Can you work these out from the model? Positions are in its coordinate system, mm. A direction names the side the tool comes from. Round coordinates to 2 decimals unless told otherwise and drop trailing zeros. Loops run counter-clockwise (first coordinate to the right, second up) from the corner with the lowest first, then second, coordinate; pieces in that order, holes last. Notation, with made-up numbers: (-21, 84.5) -> (6, 84.5) arc R3 cw to (6, 88.5) -> close; hole circle Ø11 at (74, -27). An arc over 180 degrees is marked (long way). Write each question's results on one line, items separated by ' | '.
from build123d import *

# Parameters (mm, degrees)
SKETCH1_R           = 1
SKETCH1_W           = 3
SKETCH1_H           = 5
BOSS_EXTRUDE1_DEPTH = 3


with BuildPart() as part:
    # Sketch1 → Boss-Extrude1 (new body)
    with BuildSketch(Plane.XY):
        with BuildLine():
            ThreePointArc((20, 38.729833462), (19.160374698, 38.936968749), (18.316467633, 39.125904029))
            Line((18.316467633, 39.125904029), (17.276909179, 34.235166026))
            Line((17.276909179, 34.235166026), (14.342466376, 34.858901098))
            Line((14.342466376, 34.858901098), (15.35860178, 39.639442314))
            ThreePointArc((15.35860178, 39.639442314), (12.685359142, 39.909758785), (10, 40))
            Line((10, 40), (10, 35))
            Line((10, 35), (7, 35))
            Line((7, 35), (7, 39.88734135))
            ThreePointArc((7, 39.88734135), (3.47428501, 39.464098164), (0, 38.729833462))
            Line((0, 38.729833462), (0, 0))
            Line((0, 0), (20, 0))
            Line((20, 0), (20, 38.729833462))
        make_face()
        with Locations((2.5, 2.5)):
            Circle(SKETCH1_R, mode=Mode.SUBTRACT)
        with Locations((2.5, 5.5)):
            Circle(SKETCH1_R, mode=Mode.SUBTRACT)
        with Locations((2.5, 8.5)):
            Circle(SKETCH1_R, mode=Mode.SUBTRACT)
        with Locations((5.5, 2.5)):
            Circle(SKETCH1_R, mode=Mode.SUBTRACT)
        with Locations((8.5, 2.5)):
            Circle(SKETCH1_R, mode=Mode.SUBTRACT)
        with Locations((5.5, 5.5)):
            Circle(SKETCH1_R, mode=Mode.SUBTRACT)
        with Locations((5.5, 8.5)):
            Circle(SKETCH1_R, mode=Mode.SUBTRACT)
        with Locations((8.5, 5.5)):
            Circle(SKETCH1_R, mode=Mode.SUBTRACT)
        with Locations((8.5, 8.5)):
            Circle(SKETCH1_R, mode=Mode.SUBTRACT)
        with Locations((2.5, 11.5)):
            Circle(SKETCH1_R, mode=Mode.SUBTRACT)
        with Locations((2.5, 14.5)):
            Circle(SKETCH1_R, mode=Mode.SUBTRACT)
        with Locations((2.5, 17.5)):
            Circle(SKETCH1_R, mode=Mode.SUBTRACT)
        with Locations((5.5, 11.5)):
            Circle(SKETCH1_R, mode=Mode.SUBTRACT)
        with Locations((5.5, 14.5)):
            Circle(SKETCH1_R, mode=Mode.SUBTRACT)
        with Locations((8.5, 11.5)):
            Circle(SKETCH1_R, mode=Mode.SUBTRACT)
        with Locations((8.5, 14.5)):
            Circle(SKETCH1_R, mode=Mode.SUBTRACT)
        with Locations((5.5, 17.5)):
            Circle(SKETCH1_R, mode=Mode.SUBTRACT)
        with Locations((8.5, 17.5)):
            Circle(SKETCH1_R, mode=Mode.SUBTRACT)
        with Locations((11.5, 2.5)):
            Circle(SKETCH1_R, mode=Mode.SUBTRACT)
        with Locations((14.5, 2.5)):
            Circle(SKETCH1_R, mode=Mode.SUBTRACT)
        with Locations((11.5, 5.5)):
            Circle(SKETCH1_R, mode=Mode.SUBTRACT)
        with Locations((11.5, 8.5)):
            Circle(SKETCH1_R, mode=Mode.SUBTRACT)
        with Locations((14.5, 5.5)):
            Circle(SKETCH1_R, mode=Mode.SUBTRACT)
        with Locations((14.5, 8.5)):
            Circle(SKETCH1_R, mode=Mode.SUBTRACT)
        with Locations((17.5, 2.5)):
            Circle(SKETCH1_R, mode=Mode.SUBTRACT)
        with Locations((17.5, 5.5)):
            Circle(SKETCH1_R, mode=Mode.SUBTRACT)
        with Locations((17.5, 8.5)):
            Circle(SKETCH1_R, mode=Mode.SUBTRACT)
        with Locations((11.5, 11.5)):
            Circle(SKETCH1_R, mode=Mode.SUBTRACT)
        with Locations((11.5, 14.5)):
            Circle(SKETCH1_R, mode=Mode.SUBTRACT)
        with Locations((14.5, 11.5)):
            Circle(SKETCH1_R, mode=Mode.SUBTRACT)
        with Locations((14.5, 14.5)):
            Circle(SKETCH1_R, mode=Mode.SUBTRACT)
        with Locations((11.5, 17.5)):
            Circle(SKETCH1_R, mode=Mode.SUBTRACT)
        with Locations((14.5, 17.5)):
            Circle(SKETCH1_R, mode=Mode.SUBTRACT)
        with Locations((17.5, 11.5)):
            Circle(SKETCH1_R, mode=Mode.SUBTRACT)
        with Locations((17.5, 14.5)):
            Circle(SKETCH1_R, mode=Mode.SUBTRACT)
        with Locations((17.5, 17.5)):
            Circle(SKETCH1_R, mode=Mode.SUBTRACT)
        with Locations((8.5, 22.5)):
            Rectangle(SKETCH1_W, SKETCH1_H, mode=Mode.SUBTRACT)
        Polygon((15.19779227, 24.453690018), (14.158233816, 19.562952015), (11.223791014, 20.186687087), (12.263349468, 25.077425091), align=None, mode=Mode.SUBTRACT)
    extrude(amount=BOSS_EXTRUDE1_DEPTH)


solid = part.part
1. If we section it at A-A (x = 8.5): State how many separate pieces and enclosed holes the cut face has, then the cut area to 3 significant figures.
Final values:
separate pieces: 8 | enclosed holes: 0 | area: 54.0 mm2
2. On a 3-axis mill with a long thin cutter (end or side, diameter ignored), from which of +Z, -Z, +X, -X, +Y, -Y can I reach the whole of each face in a straight line? I mean faces 1 (the face through (17.8, 36.7, 1.5)), 2 (the face through (8, 20, 1)). Say none if no direction works.
Final values:
face 1: +Z, -Z, +Y | face 2: +Z, -Z
3. Will this pin go through, and if not, where does the flat tip stop? pin 1 (1.5 mm diameter, centred on x = 5, z = 2, fed in from +Y).
Final values:
pin 1: y = 39.77
4. If we section it at D-D (y = 22.5): List the corners of the cut face in (x, z) for me.
Final values:
outline: (0, 0) -> (7, 0) -> (7, 3) -> (0, 3) -> close; (10, 0) -> (11.72, 0) -> (11.72, 3) -> (10, 3) -> close; (14.78, 0) -> (20, 0) -> (20, 3) -> (14.78, 3) -> close
5. If we section it at B-B (y = 5.5): List the corners of the cut face in (x, z) for me, then the cut area to 3 significant figures.
Final values:
outline: (0, 0) -> (1.5, 0) -> (1.5, 3) -> (0, 3) -> close; (3.5, 0) -> (4.5, 0) -> (4.5, 3) -> (3.5, 3) -> close; (6.5, 0) -> (7.5, 0) -> (7.5, 3) -> (6.5, 3) -> close; (9.5, 0) -> (10.5, 0) -> (10.5, 3) -> (9.5, 3) -> close; (12.5, 0) -> (13.5, 0) -> (13.5, 3) -> (12.5, 3) -> close; (15.5, 0) -> (16.5, 0) -> (16.5, 3) -> (15.5, 3) -> close; (18.5, 0) -> (20, 0) -> (20, 3) -> (18.5, 3) -> close | area: 24.0 mm2
6. We'd pull the mould along X, two halves only. Please class faces 3 (the face through (5.37, 9.49, 1.48)), 4 (the face through (12, 25, 3)): pulls with the +X half, pulls with the -X half, needs draft (parallel to the pull), parting line crosses it, or undercut.
Final values:
face 3: undercut | face 4: needs draft
7. If we section it at C-C (x = 2.5): List the corners of the cut face in (y, z) for me, then the cut area to 3 significant figures.
Final values:
outline: (0, 0) -> (1.5, 0) -> (1.5, 3) -> (0, 3) -> close; (3.5, 0) -> (4.5, 0) -> (4.5, 3) -> (3.5, 3) -> close; (6.5, 0) -> (7.5, 0) -> (7.5, 3) -> (6.5, 3) -> close; (9.5, 0) -> (10.5, 0) -> (10.5, 3) -> (9.5, 3) -> close; (12.5, 0) -> (13.5, 0) -> (13.5, 3) -> (12.5, 3) -> close; (15.5, 0) -> (16.5, 0) -> (16.5, 3) -> (15.5, 3) -> close; (18.5, 0) -> (39.29, 0) -> (39.29, 3) -> (18.5, 3) -> close | area: 81.9 mm2
